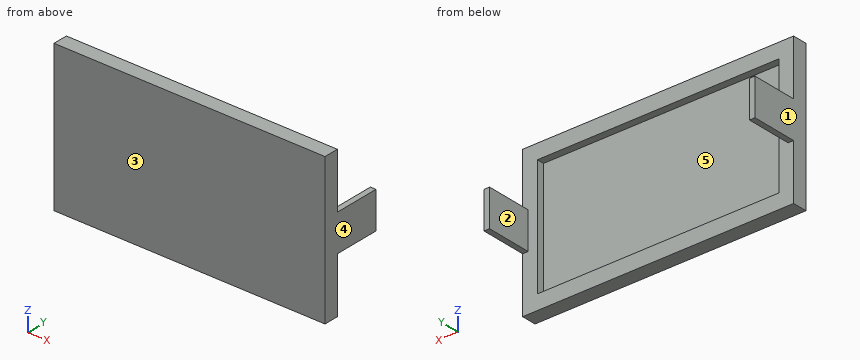
```python
from build123d import *

# Parameters (mm, degrees)
SKETCH1_W           = 147.57
SKETCH1_H           = 80.42
BOSS_EXTRUDE1_DEPTH = 8
SKETCH2_W           = 131.57
SKETCH2_H           = 64.42
CUT_EXTRUDE1_DEPTH  = 4
SKETCH3_W           = 3
SKETCH3_H           = 20
BOSS_EXTRUDE2_DEPTH = 25


with BuildPart() as part:
    # Sketch1 → Boss-Extrude1 (new body)
    with BuildSketch(Plane(origin=(0, 0, 0), x_dir=(1, 0, 0), z_dir=(0, 1, 0))):
        with Locations((73.785, 40.21)):
            Rectangle(SKETCH1_W, SKETCH1_H)
    extrude(amount=BOSS_EXTRUDE1_DEPTH)

    # Sketch2 → Cut-Extrude1 (cut)
    with BuildSketch(Plane(origin=(0, 8, 0), x_dir=(1, 0, 0), z_dir=(0, 1, 0))):
        with Locations((73.785, 40.21)):
            Rectangle(SKETCH2_W, SKETCH2_H)
    extrude(amount=-CUT_EXTRUDE1_DEPTH, mode=Mode.SUBTRACT)

    # Sketch3 → Boss-Extrude2 (add)
    with BuildSketch(Plane(origin=(0, 8, 0), x_dir=(1, 0, 0), z_dir=(0, 1, 0))):
        with Locations((1.5, 40.21)):
            Rectangle(SKETCH3_W, SKETCH3_H)
    boss_extrude2 = extrude(amount=BOSS_EXTRUDE2_DEPTH)

    # Mirror1: Boss-Extrude2 across plane
    add(boss_extrude2.mirror(Plane.ZY.offset(-73.785)))


solid = part.part
```
Geometry check sheet. Reference: the model listing, model coordinates, mm. Face numbers are marked on the shaded views. A direction names the side the tool comes from. Round coordinates to 2 decimals unless told otherwise and drop trailing zeros. Loops run counter-clockwise (first coordinate to the right, second up) from the corner with the lowest first, then second, coordinate; pieces in that order, holes last. Notation, with made-up numbers: (41, 6.25) - (87, 6.25) arc R17 cw to (87, 25.25) - close; hole circle Ø8 at (71.5, 59). An arc over 180 degrees is marked (long way). Use a Markdown table: item, result.
Q1. Draft check along X on the marked faces 1, 2 and 3. Enter one of: released by +X, released by -X, zero draft, split by the parting line, or undercut.
Solutions:
| item | result |
|---|---|
| face 1 | released by -X |
| face 2 | undercut |
| face 3 | zero draft |
Q2. Cross-section at A-A on y = 25. Record the cut outline in (x, z), plus the area to 3 significant figures.
Solutions:
| item | result |
|---|---|
| outline | (0, -50.21) - (3, -50.21) - (3, -30.21) - (0, -30.21) - close; (144.57, -50.21) - (147.57, -50.21) - (147.57, -30.21) - (144.57, -30.21) - close |
| area | 120 mm2 |
Q3. Cross-section at D-D on z = -34. Record the cut outline in (x, y), plus the area to 3 significant figures.
Solutions:
| item | result |
|---|---|
| outline | (0, 0) - (147.57, 0) - (147.57, 33) - (144.57, 33) - (144.57, 8) - (139.57, 8) - (139.57, 4) - (8, 4) - (8, 8) - (3, 8) - (3, 33) - (0, 33) - close |
| area | 804 mm2 |
Q4. Cross-section at B-B on z = -14.5. Record the cut outline in (x, y), plus the area to 3 significant figures.
Solutions:
| item | result |
|---|---|
| outline | (0, 0) - (147.57, 0) - (147.57, 8) - (139.57, 8) - (139.57, 4) - (8, 4) - (8, 8) - (0, 8) - close |
| area | 654 mm2 |
Q5. Material ranges on line 1 (X direction, y = 6, z = -17.5); line 2 (Y direction, x = 89, z = -19); line 3 (X direction, y = 27.5, z = -39.5), recorded low to high.
Solutions:
| item | result |
|---|---|
| line 1 | x = 0 to 8, 139.57 to 147.57 |
| line 2 | y = 0 to 4 |
| line 3 | x = 0 to 3, 144.57 to 147.57 |
Q6. Cross-section at C-C on x = 23.5. Record the cut outline in (y, z).
Solutions:
| item | result |
|---|---|
| outline | (0, -80.42) - (8, -80.42) - (8, -72.42) - (4, -72.42) - (4, -8) - (8, -8) - (8, 0) - (0, 0) - close |
Q7. Go/stop test with flat-tipped pins: P1, Ø3.5, axis at x = 1, y = 14.5, coming from the +Z side; P2, Ø3.5, axis at x = 145.5, y = 24.5, coming from the -Z side; P3, Ø1.5, axis at x = 47.5, z = -47.5, coming from the +Y side. Record where each tip stops, or that it passes through.
Solutions:
| item | result |
|---|---|
| P1 | stops at z = -30.21 |
| P2 | stops at z = -50.21 |
| P3 | stops at y = 4 |
Q8. Access from +Z, -Z, +X, -X, +Y, -Y to the whole of each face (thin tool, end or side, straight path). Record for the marked faces 4 and 5.
Solutions:
| item | result |
|---|---|
| face 4 | +Z, -Z, +X, +Y, -Y |
| face 5 | +Y |
